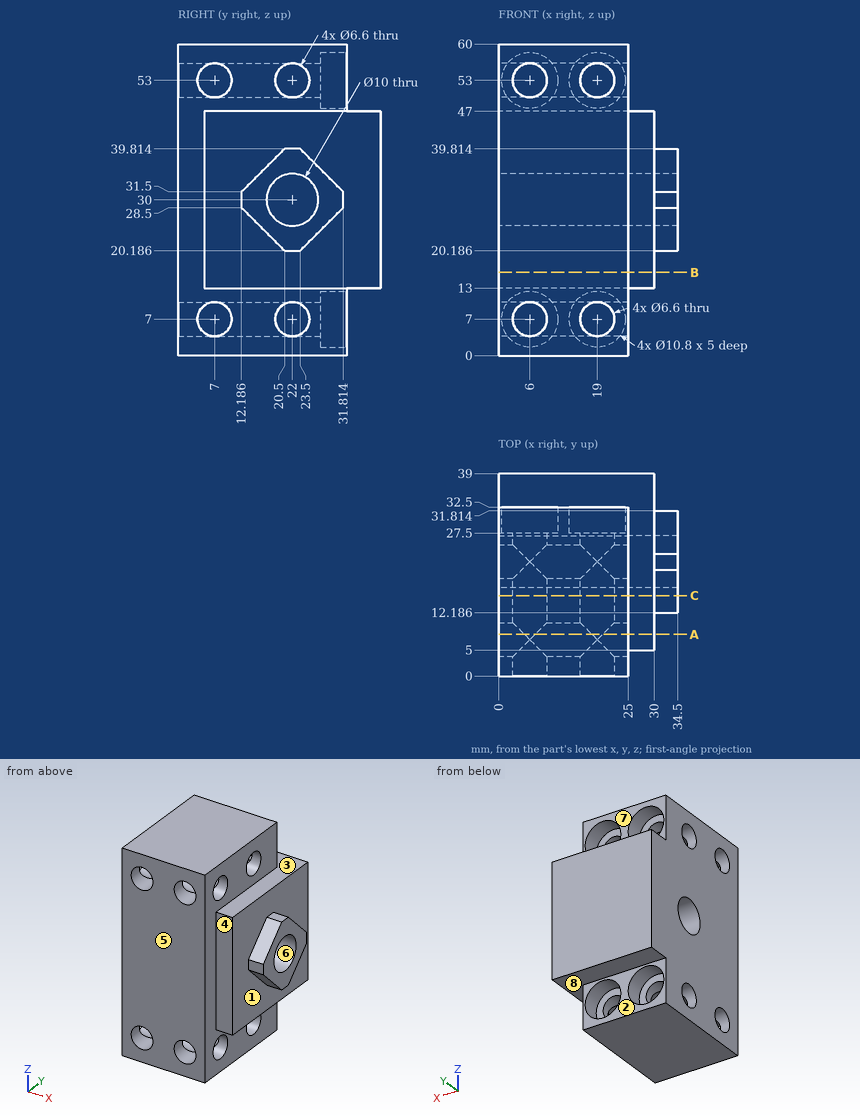
For this review, use the dimensioned drawing (mm, ordinates from the lowest corner) and the shaded views. A direction names the side the tool comes from. Round coordinates to 2 decimals unless told otherwise and drop trailing zeros. Loops run counter-clockwise (first coordinate to the right, second up) from the corner with the lowest first, then second, coordinate; pieces in that order, holes last. Notation, with made-up numbers: M 65.5,-33.5 L 70.5,-33.5 A19 ccw 70.5,-0.5 Z; hole C 28,1.5 d8. An arc over 180 degrees is marked long. Answer as a JSON object with one key per item and string values.
(1) Take a section at B-B on z = 16. Give the boundary of the cut face in (x, y), and give its area (4 significant figures).
Resolved:
{"outline": "M 0,0 L 25,0 L 25,5 L 30,5 L 30,39 L 0,39 Z", "area": "1,145 mm²"}
(2) Tool access review of the marked faces 1, 2, 3 and 4: name each direction out of +Z, -Z, +X, -X, +Y, -Y from which nothing blocks a thin tool from reaching the whole face with its end or side.
Resolved:
{"face 1": "+X", "face 2": "-Z, +X, -X, +Y", "face 3": "+Z, +X, +Y", "face 4": "+Z, -Z, +X, -Y"}
(3) Take a section at C-C on y = 15.5. Give the boundary of the cut face in (x, z), and give its area (3 significant figures).
Resolved:
{"outline": "M 0,0 L 25,0 L 25,13 L 30,13 L 30,25.19 L 34.5,25.19 L 34.5,34.81 L 30,34.81 L 30,47 L 25,47 L 25,60 L 0,60 Z; hole C 6,7 d6.6; hole C 6,53 d6.6; hole C 19,7 d6.6; hole C 19,53 d6.6", "area": "1,580 mm²"}
(4) Draft analysis for pull direction Y (two halves, no side actions). For the marked faces 5, 6, 7 and 8, state which applies: released by +Y, released by -Y, zero draft, split by the parting line, or undercut.
Resolved:
{"face 5": "released by -Y", "face 6": "undercut", "face 7": "released by +Y", "face 8": "zero draft"}
(5) To check wall thickness, follow line 1 along X through (y, z) = (2.5, 53); line 2 along Z through (x, y) = (19, 4); line 3 along X through (y, z) = (30, 7). State the ranges of each line that lie inside material, in increasing order.
Resolved:
{"line 1": "0 to 2.7, 9.3 to 15.7, 22.3 to 25", "line 2": "0 to 3.7, 10.3 to 49.7, 56.3 to 60", "line 3": "0 to 0.6, 11.4 to 13.6, 24.4 to 25"}
(6) Take a section at A-A on y = 8. Count the separate pieces of the cut face and the enclosed holes in it, and give its area (3 significant figures).
Resolved:
{"separate pieces": "3", "enclosed holes": "0", "area": "1,350 mm²"}
(7) Clearance check with flat-ended pins moving along their axes: P1, Ø4, axis at x = 25.5, y = 19, coming from the +Z side; P2, Ø2.5, axis at x = 31.5, z = 29.5, coming from the -Y side; P3, Ø6, axis at y = 7, z = 7, coming from the -X side; P4, Ø9.5, axis at x = 19, z = 7, coming from the +Y side. State where each tip first meets the part, or that it passes through.
Resolved:
{"P1": "z = 60", "P2": "y = 12.19", "P3": "through", "P4": "y = 27.5"}
